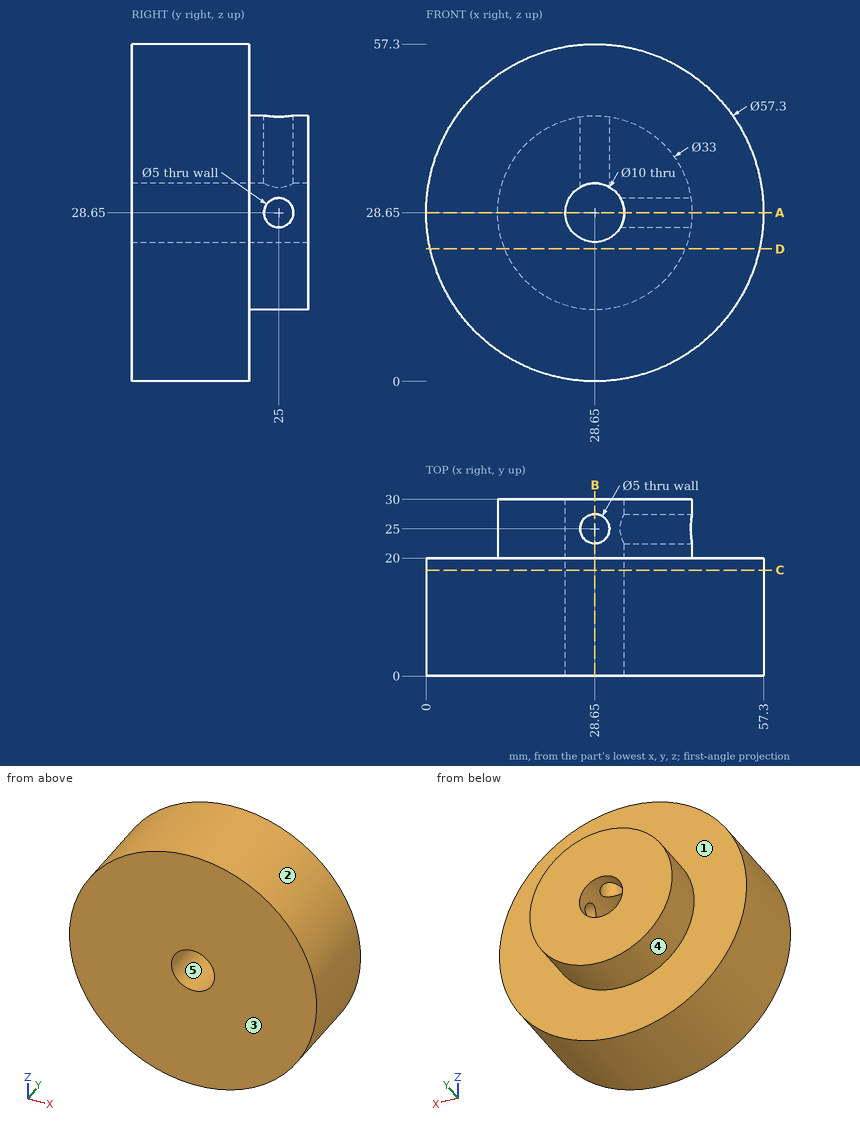
Check sheet for the drawn part. Datum: minimum x, y, z corner. Units: mm. A direction names the side the tool comes from. Give positions to 0.01 mm unless a question says otherwise; leave off trailing zeros. Write each loop counter-clockwise with the first axis right and the second up, starting at its lowest first coordinate (ties: lowest second). Pieces come first, ordered by that corner, then holes. Notation, with made-up numbers: M 56,52 L 110,52 A8 ccw 110,56 Z; hole C -36,75 d3. An arc over 180 degrees is marked long. Write item = value, one per line.
(1) Material ranges on line 1 (Y direction, x = 42.5, z = 28.65); line 2 (Y direction, x = 25, z = 45); line 3 (X direction, y = 18.5, z = 31), recorded low to high.
Found:
line_1 = 0 to 22.5, 27.5 to 30
line_2 = 0 to 20
line_3 = 0.1 to 24.24, 33.06 to 57.2
(2) Draft check along Z on the marked faces 3, 4 and 5. Enter one of: released by +Z, released by -Z, zero draft, split by the parting line, or undercut.
Found:
face_3 = zero draft
face_4 = split by the parting line
face_5 = undercut
(3) Sectioned sample at C-C (y = 18). Record the cut outline in (x, z), then the cut area to 3 significant figures.
Found:
outline = C 28.65,28.65 d57.3; hole C 28.65,28.65 d10
area = 2,500 mm2
(4) Sectioned sample at B-B (x = 28.65). Record the cut outline in (y, z).
Found:
outline = M 0,0 L 20,0 L 20,12.15 L 30,12.15 L 30,23.65 L 0,23.65 Z; M 0,33.65 L 22.5,33.65 L 22.5,45.15 L 20,45.15 L 20,57.3 L 0,57.3 Z; M 27.5,33.65 L 30,33.65 L 30,45.15 L 27.5,45.15 Z
(5) Go/stop test with flat-tipped pins: pin 1 Ø6 at (x, z) = (6, 29.5) entering from +Y; pin 2 Ø1.5 at (y, z) = (24.5, 20.5) entering from +X; pin 3 Ø10 at (x, y) = (22, 9) entering from +Z. Record where each tip stops, or that it passes through.
Found:
pin_1 = 20
pin_2 = 43.4
pin_3 = 57.25
(6) Sectioned sample at A-A (z = 28.65). Record the cut outline in (x, y).
Found:
outline = M 0,0 L 23.65,0 L 23.65,30 L 12.15,30 L 12.15,20 L 0,20 Z; M 33.65,0 L 57.3,0 L 57.3,20 L 45.15,20 L 45.15,22.5 L 33.65,22.5 Z; M 33.65,27.5 L 45.15,27.5 L 45.15,30 L 33.65,30 Z
(7) Sectioned sample at D-D (z = 22.5). Record the cut outline in (x, y), then the cut area to 3 significant figures.
Found:
outline = M 0.67,0 L 56.63,0 L 56.63,20 L 43.96,20 L 43.96,30 L 13.34,30 L 13.34,20 L 0.67,20 Z
area = 1,430 mm2
(8) Access from +Z, -Z, +X, -X, +Y, -Y to the whole of each face (thin tool, end or side, straight path). Record for the marked faces 1 and 2.
Found:
face_1 = +Y
face_2 = +Y, -Y
